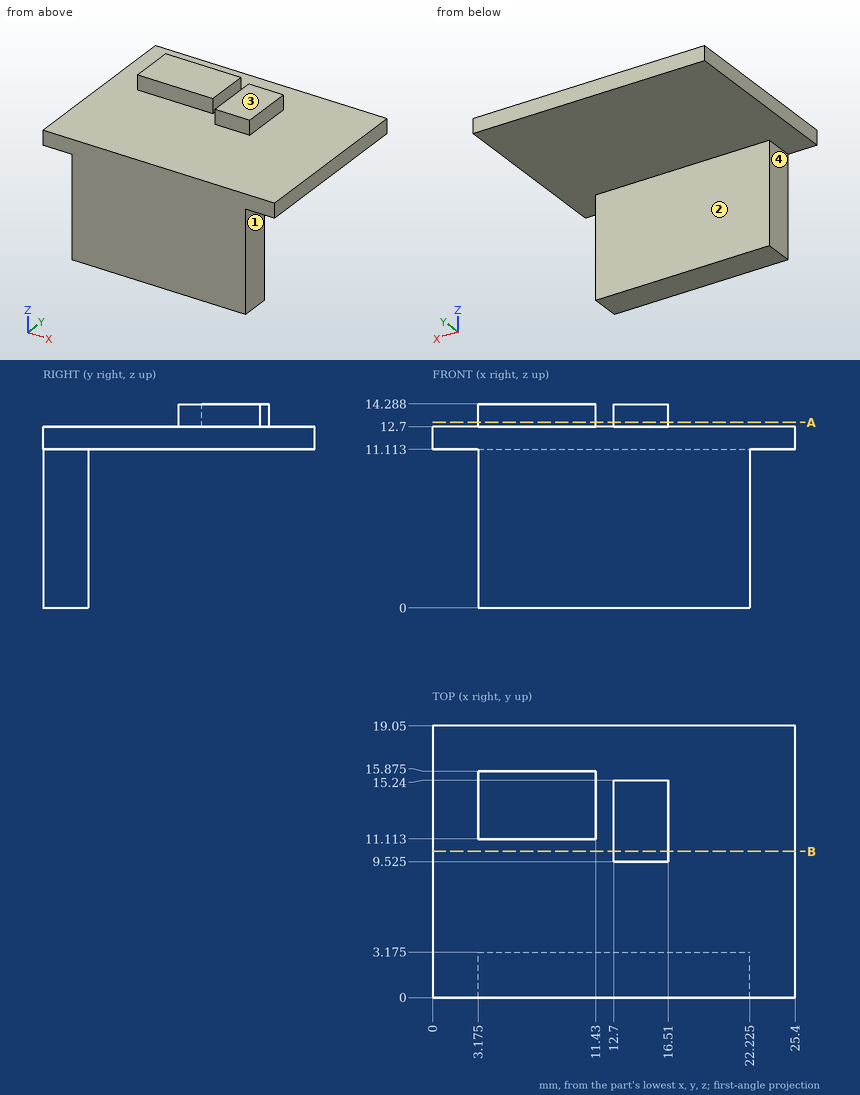
Input: dimensioned drawing with shaded views. Units: mm. Origin: part minimum x, y, z. A direction names the side the tool comes from. Round coordinates to 2 decimals unless told otherwise and drop trailing zeros. Order: outer loops, then holes, each group sorted by start corner. A loop starts at its lowest first (then second) coordinate and runs counter-clockwise, first axis right, second up. Notation, with made-up numbers: (3.25, 67) -> (59.25, 67) arc R18 ccw to (59.25, 88) -> close; hole circle Ø6 at (14.25, -34.5). An arc over 180 degrees is marked (long way). One line per item, written item: value. Start each with the question number.
Q1. Section query B-B (y = 10.25). Return the cut outline in (x, z).
Q2. Material intervals for probe 1 along X at (y, z) = (13.25, 13.25) (1 decimal); probe 2 along Z at (x, y) = (16, 3.75); probe 3 along Y at (x, z) = (17, 10.25) (1 decimal), sorted ascending.
Q3. Pin query (flat end, axial travel): pin 1 (5 mm diameter, centred on y = 3.5, z = 2.5, fed in from +X) (1 decimal); pin 2 (5 mm diameter, centred on x = 10.5, z = 12, fed in from -Y); pin 3 (1.6 mm diameter, centred on y = 1.5, z = 7.5, fed in from -X) (1 decimal); pin 4 (4 mm diameter, centred on x = 21.5, y = 11.5, fed in from -Z). Return the tip coordinate at first contact, or that it passes through.
Q4. Section query A-A (z = 13). Return the cut outline in (x, y) (1 decimal).
Q5. Access query for the marked faces 1, 2, 3 and 4. Directions: +Z, -Z, +X, -X, +Y, -Y. A direction counts if a zero-diameter tool reaches every point of the face in a straight line with its end or side. Return the directions, or none.
Findings below:
1. outline: (0, 11.11) -> (25.4, 11.11) -> (25.4, 12.7) -> (16.51, 12.7) -> (16.51, 14.29) -> (12.7, 14.29) -> (12.7, 12.7) -> (0, 12.7) -> close
2. probe 1: 3.2 to 11.4, 12.7 to 16.5
2. probe 2: 11.11 to 12.7
2. probe 3: 0 to 3.2
3. pin 1: x = 22.2
3. pin 2: y = 0
3. pin 3: x = 3.2
3. pin 4: z = 11.11
4. outline: (3.2, 11.1) -> (11.4, 11.1) -> (11.4, 15.9) -> (3.2, 15.9) -> close; (12.7, 9.5) -> (16.5, 9.5) -> (16.5, 15.2) -> (12.7, 15.2) -> close
5. face 1: -Z, +X, +Y, -Y
5. face 2: -Z, +X, -X, +Y
5. face 3: +Z, +X, -X, +Y, -Y
5. face 4: -Z, -X, +Y, -Y
